```python
from build123d import *

# Parameters (mm, degrees)
BASPROSKE_W        = 4
BASPROSKE_H        = 14
TOOTHCUT_DEPTH     = 21.199009877
TEETHCUTS_COUNT    = 26
TEETHCUTS_ANGLE    = 346.153846154
BORSKE_R           = 3
BORE_DEPTH         = 50.0000508
HOLE_WIZARD_M3_1_D = 3.4
CIRPATTERN1_COUNT  = 4


with BuildPart() as part:
    # BasProSke → Base-Revolve (revolve)
    with BuildSketch(Plane(origin=(0, 0, 0), x_dir=(1, 0, 0), z_dir=(0, 1, 0)), mode=Mode.PRIVATE) as base_revolve_sk:
        with Locations((2, 7)):
            Rectangle(BASPROSKE_W, BASPROSKE_H)
    revolve(base_revolve_sk.sketch.rotate(Axis((-10, 0, 0), (1, 0, 0)), 180), axis=Axis((-10, 0, 0), (1, 0, 0)))

    # TooCutSke → ToothCut (cut, through all)
    with BuildSketch(Plane(origin=(0, 0, 0), x_dir=(0, 0, -1), z_dir=(1, 0, 0))):
        with BuildLine():
            ThreePointArc((0.476965065, 11.739314517), (0, 11.749), (-0.476965065, 11.739314517))
            ThreePointArc((-0.476965065, 11.739314517), (-0.82065865, 12.901686978), (-1.424117301, 13.952911348))
            ThreePointArc((-1.424117301, 13.952911348), (0, 14.0254), (1.424117301, 13.952911348))
            ThreePointArc((1.424117301, 13.952911348), (0.82065865, 12.901686978), (0.476965065, 11.739314517))
        make_face()
    toothcut = extrude(amount=TOOTHCUT_DEPTH, mode=Mode.SUBTRACT)

    # TeethCuts: ToothCut ×26 about axis
    teethcuts_axis = Axis((-10, 0, 0), (1, 0, 0))
    for i in range(1, TEETHCUTS_COUNT):
        add(toothcut.rotate(teethcuts_axis, i * TEETHCUTS_ANGLE / (TEETHCUTS_COUNT - 1)), mode=Mode.SUBTRACT)

    # BorSke → Bore (cut, symmetric)
    with BuildSketch(Plane(origin=(0, 0, 0), x_dir=(0, 0, -1), z_dir=(1, 0, 0))):
        with Locations(Location((0, 0, 0), (0, 0, 180))):
            Circle(BORSKE_R)
    extrude(amount=BORE_DEPTH, both=True, mode=Mode.SUBTRACT)

    # M3 餘隙孔1 (through all)
    with Locations(Plane(origin=(4, 0, 0), x_dir=(0, 0, -1), z_dir=(1, 0, 0))):
        with Locations((0, 7)):
            hole_wizard_m3_1 = Hole(HOLE_WIZARD_M3_1_D / 2)

    # CirPattern1: M3 餘隙孔1 ×4 about axis
    cirpattern1_axis = Axis((0, 0, 0), (1, 0, 0))
    for i in range(1, CIRPATTERN1_COUNT):
        add(hole_wizard_m3_1.rotate(cirpattern1_axis, i * 360 / CIRPATTERN1_COUNT), mode=Mode.SUBTRACT)


solid = part.part
```
Input: part model. Units: mm. Frame: model coordinates. A direction names the side the tool comes from. Round coordinates to 2 decimals unless told otherwise and drop trailing zeros. Write each loop counter-clockwise with the first axis right and the second up, starting at its lowest first coordinate (ties: lowest second). Pieces come first, ordered by that corner, then holes. Notation, with made-up numbers: (13.5, 49) - (26.5, 49) arc R22 cw to (26.5, 64) - close; hole circle Ø10 at (-1.75, 49). An arc over 180 degrees is marked (long way). Write item = value, one per line.
(1) Section query C-C on x = 0.55. State how many separate pieces and enclosed holes the cut face has, then the cut area to 3 significant figures.
Geometry check:
separate_pieces = 1
enclosed_holes = 5
area = 452 mm^2
(2) Pull-direction query (Z, two-part tool) for faces 4 (the cylindrical face through (1.972, 8.006, 10.153)), 5 (the cylindrical face through (1.97, -0.75, -12.88)), 6 (the cylindrical face through (1.972, -6.654, 11.086)); classes: +Z half, -Z half, draft (parallel to the pull), parting line (faces both ways), or undercut.
Geometry check:
face_4 = +Z half
face_5 = -Z half
face_6 = undercut
(3) Material intervals for probe 1 along Y at (x, z) = (2.6, 0); probe 2 along Y at (x, z) = (2.35, 12); probe 3 along Y at (x, z) = (1.5, -1.25), sorted ascending.
Geometry check:
probe_1 = -11.75 to -8.7, -5.3 to -3, 3 to 5.3, 8.7 to 11.75
probe_2 = -6.76 to -5.58, -3.81 to -2.03, -0.92 to 0.92, 2.03 to 3.81, 5.58 to 6.76
probe_3 = -13.7 to -8.15, -5.85 to -2.73, 2.73 to 5.85, 8.15 to 13.7
(4) Section query A-A on z = 0. Output: boundary loops of the cut face in (x, y), then the cut area to 3 significant figures.
Geometry check:
outline = (0, -11.75) - (4, -11.75) - (4, -8.7) - (0, -8.7) - close; (0, -5.3) - (4, -5.3) - (4, -3) - (0, -3) - close; (0, 3) - (4, 3) - (4, 5.3) - (0, 5.3) - close; (0, 8.7) - (4, 8.7) - (4, 11.75) - (0, 11.75) - close
area = 42.8 mm^2
(5) Section query B-B on z = -7. Output: boundary loops of the cut face in (x, y), then the cut area to 3 significant figures.
Geometry check:
outline = (0, -11.25) - (4, -11.25) - (4, -1.7) - (0, -1.7) - close; (0, 1.7) - (4, 1.7) - (4, 11.25) - (0, 11.25) - close
area = 76.4 mm^2
(6) Contact query for flat-ended pins moving along their axis: pin 1 Ø2 at (x, y) = (2.5, -3.5) entering from -Z; pin 2 Ø1.5 at (x, z) = (2, -3.5) entering from +Y; pin 3 Ø1.5 at (x, y) = (1.5, -2.5) entering from +Z. Output: stop coordinate, or through.
Geometry check:
pin_1 = -13.66
pin_2 = 12.76
pin_3 = 13.66
(7) Access query for faces 1 (the cylindrical face through (1.97, 5.32, -11.75)), 2 (the cylindrical face through (1.97, 5.34, 11.77)), 3 (the cylindrical face through (1.97, 11.81, 5.27)). Directions: +Z, -Z, +X, -X, +Y, -Y. A direction counts if a zero-diameter tool reaches every point of the face in a straight line with its end or side. Return the directions, or none.
Geometry check:
face_1 = -Z, +X, -X
face_2 = +Z, +X, -X
face_3 = +X, -X
